from build123d import *

# Parameters (mm, degrees)
ESQUISSE1_R                  = 2
ESQUISSE1_R_2                = 2.5
BOSS_EXTRU_1_DEPTH           = 5.5
ESQUISSE2_W                  = 3
ESQUISSE2_H                  = 10
ENL_V_MAT_EXTRU_1_DEPTH      = 5
ENL_V_MAT_EXTRU_1_DEPTH_BACK = 5


with BuildPart() as part:
    # Esquisse1 → Boss.-Extru.1 (new body)
    with BuildSketch(Plane.XY):
        with BuildLine():
            Line((-4, -7), (-4, 7))
            ThreePointArc((-4, 7), (0, 11), (4, 7))
            Line((4, 7), (4, -7))
            ThreePointArc((4, -7), (0, -11), (-4, -7))
        make_face()
        with Locations((0, -7)):
            Circle(ESQUISSE1_R, mode=Mode.SUBTRACT)
        with Locations((0, 7)):
            Circle(ESQUISSE1_R_2, mode=Mode.SUBTRACT)
    extrude(amount=BOSS_EXTRU_1_DEPTH)

    # Esquisse2 → Enlèv. mat.-Extru.1 (cut, two sides)
    with BuildSketch(Plane(origin=(0, 0, 0), x_dir=(0, 0, -1), z_dir=(1, 0, 0))) as enl_v_mat_extru_1_sk:
        with Locations((-1.5, 6)):
            Rectangle(ESQUISSE2_W, ESQUISSE2_H)
    extrude(amount=ENL_V_MAT_EXTRU_1_DEPTH, mode=Mode.SUBTRACT)
    extrude(enl_v_mat_extru_1_sk.sketch, amount=-ENL_V_MAT_EXTRU_1_DEPTH_BACK, mode=Mode.SUBTRACT)


solid = part.part
Can you work these out from the model? Positions are in its coordinate system, mm. A direction names the side the tool comes from. Coordinates: 2 decimals unless noted, no trailing zeros. Order: outer loops, then holes, each group sorted by start corner. A loop starts at its lowest first (then second) coordinate and runs counter-clockwise, first axis right, second up. Notation, with made-up numbers: M 73,83.25 L 97,83.25 A12 ccw 97,99.25 Z; hole C 59,-35 d3. An arc over 180 degrees is marked long. Write item = value, one per line.
(1) If we mould it in two halves opening along Y, with no side actions, what happens to faces 3 (the face through (0, -11, 3)), 4 (the face through (1.908, -6.399, 2.712)), 5 (the face through (-4, -2, 3))? For each: pulls with the +Y half, pulls with the -Y half, needs draft (parallel to the pull), parting line crosses it, or undercut.
Results are:
face_3 = pulls with the -Y half
face_4 = undercut
face_5 = needs draft
(2) Suppose I cut it at D-D on z = 2.35. Please give me the cut outline in (x, y), plus the area to 3 significant figures.
Results are:
outline = M -4,-7 A4 ccw 4,-7 L 4,1 L -4,1 Z; hole C 0,-7 d4
area = 76.6 mm2
(3) Suppose I cut it at A-A on x = 0. Please give me the cut outline in (y, z).
Results are:
outline = M -11,0 L -9,0 L -9,5.5 L -11,5.5 Z; M -5,0 L 1,0 L 1,3 L 4.5,3 L 4.5,5.5 L -5,5.5 Z; M 9.5,3 L 11,3 L 11,5.5 L 9.5,5.5 Z
(4) Suppose I cut it at B-B on y = -6. Please give me the cut outline in (x, z), plus the area to 3 significant figures.
Results are:
outline = M -4,0 L -1.73,0 L -1.73,5.5 L -4,5.5 Z; M 1.73,0 L 4,0 L 4,5.5 L 1.73,5.5 Z
area = 24.9 mm2
(5) For faces 1 (the face through (0, 1, 2)), 2 (the face through (0, 0, 5.5)), which set-ups out of +Z, -Z, +X, -X, +Y, -Y let a thin tool reach every point of the face, with its end or its side?
Results are:
face_1 = -Z, +X, -X, +Y
face_2 = +Z, +X, -X, +Y, -Y
(6) I need wall thicknesses on line 1 along Y through (x, z) = (0, 4.1); line 2 along Y through (x, z) = (-1.75, 4.75); line 3 along Z through (x, y) = (1.5, 1.25). Which ranges of each line are inside material? Lowest first, please. Write a range as [from, to].
Results are:
line_1 = [-11, -9], [-5, 4.5], [9.5, 11]
line_2 = [-10.6, -7.97], [-6.03, 5.21], [8.79, 10.6]
line_3 = [3, 5.5]
(7) For pin 1 Ø0.9 at (x, z) = (-1, 1) entering from +Y; pin 2 Ø3 at (x, y) = (0, -7) entering from -Z, each with a flat end and sliding along its axis, tell me the tip position at first contact or that it passes through.
Results are:
pin_1 = 1
pin_2 = through
(8) Suppose I cut it at C-C on z = 4.2. Please give me the cut outline in (x, y).
Results are:
outline = M -4,-7 A4 ccw 4,-7 L 4,7 A4 ccw -4,7 Z; hole C 0,7 d5; hole C 0,-7 d4
